Here's the drawing with two shaded views (mm, measured from the low corner). I have some questions. Coordinates: 2 decimals unless noted, no trailing zeros. Write each loop counter-clockwise with the first axis right and the second up, starting at its lowest first coordinate (ties: lowest second). Pieces come first, ordered by that corner, then holes. Notation, with made-up numbers: (77.5, 80) -> (90.5, 80) arc R26 ccw to (90.5, 106) -> close; hole circle Ø3 at (45, 41). An arc over 180 degrees is marked (long way). Put each result on its own line as item: value. Start each with the question number.
Item 1: I want a section at A-A, the plane z = 9. State how many separate pieces and enclosed holes the cut face has, then the cut area to 3 significant figures.
Item 2: I want a section at B-B, the plane y = 13.8. List the corners of the cut face in (x, z) for me.
Item 3: I need wall thicknesses on line 1 (Z direction, x = 2.05, y = 34.8); line 2 (Z direction, x = 0.3, y = 26.5); line 3 (Y direction, x = 0.7, z = 7.25). Which ranges of each line are inside material? Lowest first, please. Write a range as [from, to].
Item 4: For pin 1 (0.6 mm diameter, centred on y = 78.5, z = 14, fed in from +X); pin 2 (2 mm diameter, centred on x = 1.5, y = 11.5, fed in from -Z), each with a flat end and sliding along its axis, tell me the tip position at first contact or that it passes through.
Item 5: I want a section at C-C, the plane z = 2.5. List the corners of the cut face in (x, y) for me, then the cut area to 3 significant figures.
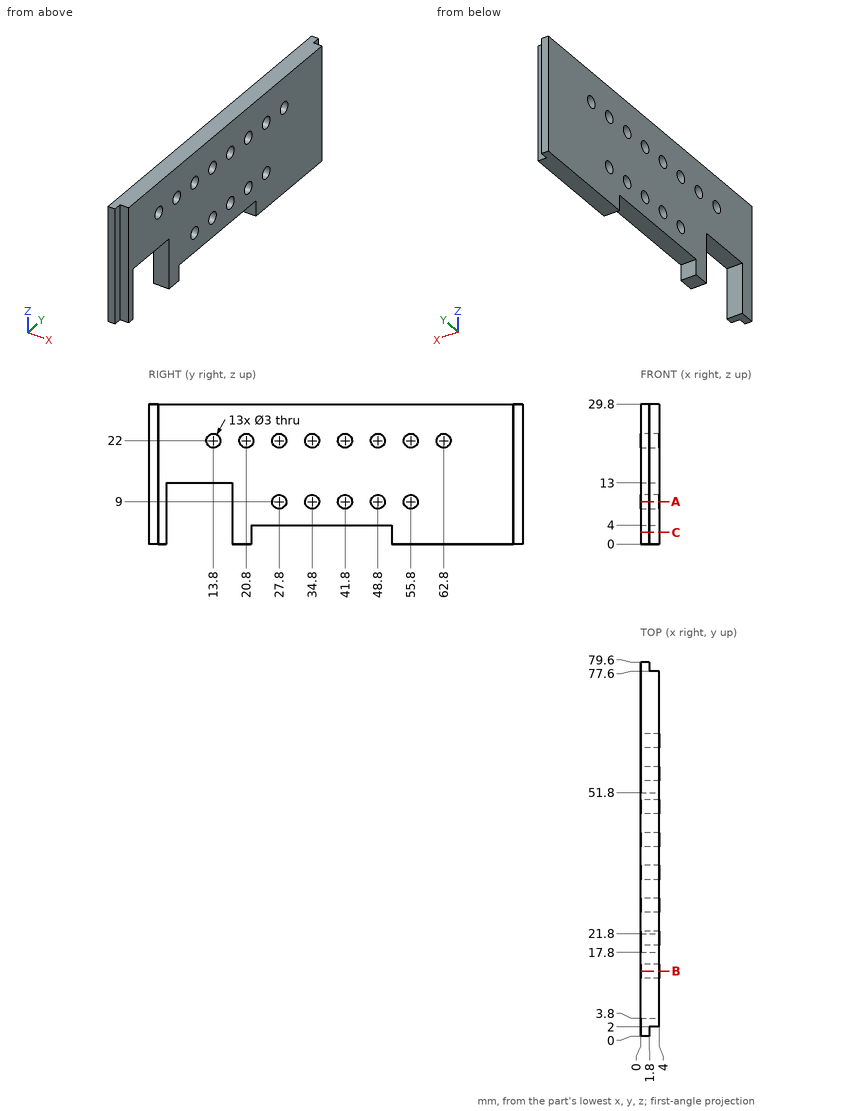
Calculated:
1. separate pieces: 7
1. enclosed holes: 0
1. area: 194 mm2
2. outline: (0, 13) -> (4, 13) -> (4, 20.5) -> (0, 20.5) -> close; (0, 23.5) -> (4, 23.5) -> (4, 29.8) -> (0, 29.8) -> close
3. line 1: z = [4, 7.5], [10.5, 20.5], [23.5, 29.8]
3. line 2: z = [4, 8.25], [9.75, 21.25], [22.75, 29.8]
3. line 3: y = [0, 3.8], [17.8, 79.6]
4. pin 1: stops at x = 1.8
4. pin 2: stops at z = 13
5. outline: (0, 0) -> (1.8, 0) -> (1.8, 2) -> (4, 2) -> (4, 3.8) -> (0, 3.8) -> close; (0, 17.8) -> (4, 17.8) -> (4, 21.8) -> (0, 21.8) -> close; (0, 51.8) -> (4, 51.8) -> (4, 77.6) -> (1.8, 77.6) -> (1.8, 79.6) -> (0, 79.6) -> close
5. area: 134 mm2
